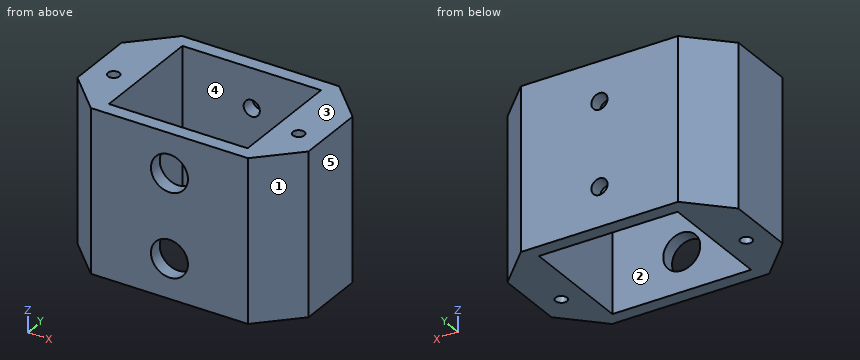
from build123d import *

# Parameters (mm, degrees)
F0_W           = 50
F0_H           = 31
F0_W_2         = 30
F0_H_2         = 25
F1_DEPTH       = 35
F3_D           = 3.5
F3_CBORE_D     = 8
F3_CBORE_DEPTH = 5
F5_D           = 2.5
F6_SIZE        = 8


with BuildPart() as f1:
    # F0 (on Top) → F1 (new body)
    with BuildSketch(Plane.XY):
        Rectangle(F0_W, F0_H)
        Rectangle(F0_W_2, F0_H_2, mode=Mode.SUBTRACT)
    extrude(amount=F1_DEPTH)

    # F3 (through all)
    with Locations(Plane.XZ.offset(15.5)):
        with Locations((0, 26.5), (0, 8.5)):
            CounterBoreHole(F3_D / 2, F3_CBORE_D / 2, F3_CBORE_DEPTH)

    # F5 (through all)
    with Locations(Plane(origin=(0, 0, 0), x_dir=(1, 0, 0), z_dir=(0, 0, -1))):
        with Locations((-20, 3), (20, 3)):
            Hole(F5_D / 2)

    # F6
    f6_edges = [f1.edges().sort_by_distance(p)[0] for p in [
        (25, -15.5, 17.5),
        (-25, -15.5, 17.5),
        (-25, 15.5, 17.5),
        (25, 15.5, 17.5),
    ]]
    chamfer(f6_edges, length=F6_SIZE)


solid = f1.part
Could you check a few things on this model? Use its own coordinates, in mm. Face numbers are marked on the shaded views. A direction names the side the tool comes from. Give positions to 0.01 mm unless a question says otherwise; leave off trailing zeros. Order: outer loops, then holes, each group sorted by start corner. A loop starts at its lowest first (then second) coordinate and runs counter-clockwise, first axis right, second up. Notation, with made-up numbers: (17, -21) - (68, -21) arc R17 ccw to (68, -9) - close; hole circle Ø3 at (-9, -35.5). An arc over 180 degrees is marked (long way). One line per item, written item: value. Start each with the question number.
1. Thinking about a two-plate mould opening in X: for the marked faces 1, 2 and 3, which applies, +X half, -X half, draft (parallel to the pull), parting line (faces both ways), or undercut?
2. For the marked faces 4 and 5, which set-ups out of +Z, -Z, +X, -X, +Y, -Y let a thin tool reach every point of the face, with its end or its side?
3. If I drill on probe 1 along Z at (x, y) = (0, 13); probe 2 along Y at (x, z) = (-6, 20); probe 3 along X at (y, z) = (-7, 2), over which ranges is the centre line in solid material (lowest first)?
4. For P1, Ø3, axis at y = 10.5, z = 20.5, coming from the -X side; P2, Ø1, axis at x = 19.5, z = 12, coming from the +Y side; P3, Ø2, axis at x = -20, y = -3, coming from the -Z side; P4, Ø6.5, axis at x = 0, z = 26.5, coming from the -Y side, each with a flat end and sliding along its axis, tell me the tip position at first contact or that it passes through.
5. Imagine slicing it at D-D on y = -9.5. List the corners of the cut face in (x, z) for me, plus the area to 3 significant figures.
6. Imagine slicing it at B-B on y = -3. List the corners of the cut face in (x, z) for me, plus the area to 3 significant figures.
7. Imagine slicing it at A-A on z = 8.5. List the corners of the cut face in (x, y) for me, plus the area to 3 significant figures.
8. Imagine slicing it at C-C on x = -20. List the corners of the cut face in (y, z) for me, plus the area to 4 significant figures.
Values:
1. face 1: +X half
1. face 2: undercut
1. face 3: draft
2. face 4: +Z, -Z
2. face 5: +Z, -Z, +X, +Y, -Y
3. probe 1: 0 to 6.75, 10.25 to 24.75, 28.25 to 35
3. probe 2: -15.5 to -12.5, 12.5 to 15.5
3. probe 3: -25 to -15, 15 to 25
4. P1: x = -23.5
4. P2: y = 13.5
4. P3: through
4. P4: y = 12.5
5. outline: (-23, 0) - (-15, 0) - (-15, 35) - (-23, 35) - close; (15, 0) - (23, 0) - (23, 35) - (15, 35) - close
5. area: 560 mm²
6. outline: (-25, 0) - (-21.25, 0) - (-21.25, 35) - (-25, 35) - close; (-18.75, 0) - (-15, 0) - (-15, 35) - (-18.75, 35) - close; (15, 0) - (18.75, 0) - (18.75, 35) - (15, 35) - close; (21.25, 0) - (25, 0) - (25, 35) - (21.25, 35) - close
6. area: 525 mm²
7. outline: (-25, -7.5) - (-17, -15.5) - (-4, -15.5) - (-4, -12.5) - (-15, -12.5) - (-15, 12.5) - (-1.75, 12.5) - (-1.75, 15.5) - (-17, 15.5) - (-25, 7.5) - close; (1.75, 12.5) - (15, 12.5) - (15, -12.5) - (4, -12.5) - (4, -15.5) - (17, -15.5) - (25, -7.5) - (25, 7.5) - (17, 15.5) - (1.75, 15.5) - close; hole circle Ø2.5 at (-20, -3); hole circle Ø2.5 at (20, -3)
7. area: 628 mm²
8. outline: (-12.5, 0) - (-4.25, 0) - (-4.25, 35) - (-12.5, 35) - close; (-1.75, 0) - (12.5, 0) - (12.5, 35) - (-1.75, 35) - close
8. area: 787.5 mm²
